```python
from build123d import *

# Parameters (mm, degrees)
BOSS_EXTRUDE1_DEPTH      = 266.7
BOSS_EXTRUDE1_DEPTH_BACK = 266.7
SKETCH3_W                = 25.4
SKETCH3_H                = 25.4
SKETCH3_W_2              = 19.05
SKETCH3_H_2              = 19.05
SKETCH4_R                = 9.525
CUT_EXTRUDE1_DEPTH       = 25.4
SKETCH5_R                = 9.525
CUT_EXTRUDE2_DEPTH       = 3.175


with BuildPart() as part:
    # Sketch3 → Boss-Extrude1 (new, two sides: drawn at the far end of the back side and taken through both)
    with BuildSketch(Plane.XY.offset(-BOSS_EXTRUDE1_DEPTH_BACK)):
        Rectangle(SKETCH3_W, SKETCH3_H)
        Rectangle(SKETCH3_W_2, SKETCH3_H_2, mode=Mode.SUBTRACT)
    extrude(amount=BOSS_EXTRUDE1_DEPTH + BOSS_EXTRUDE1_DEPTH_BACK)

    # Sketch4 → Cut-Extrude1 (cut)
    with BuildSketch(Plane(origin=(0, 12.7, 0), x_dir=(1, 0, 0), z_dir=(0, 1, 0))):
        with Locations(Location((0, 212.725, 0), (0, 0, 180))):
            Circle(SKETCH4_R)
        Polygon((-12.7, 225.013453558), (-12.7, 266.7), (12.7, 266.7), (12.7, 252.73), (-3.69434815, 252.73), align=None)
    extrude(amount=-CUT_EXTRUDE1_DEPTH, mode=Mode.SUBTRACT)

    # Sketch5 → Cut-Extrude2 (cut)
    with BuildSketch(Plane.XZ.offset(-12.7)):
        with Locations(Location((-0.660548484, -179.870948658, 0), (0, 0, 201.463465423))):
            Circle(SKETCH5_R)
    extrude(amount=CUT_EXTRUDE2_DEPTH, mode=Mode.SUBTRACT)


solid = part.part
```
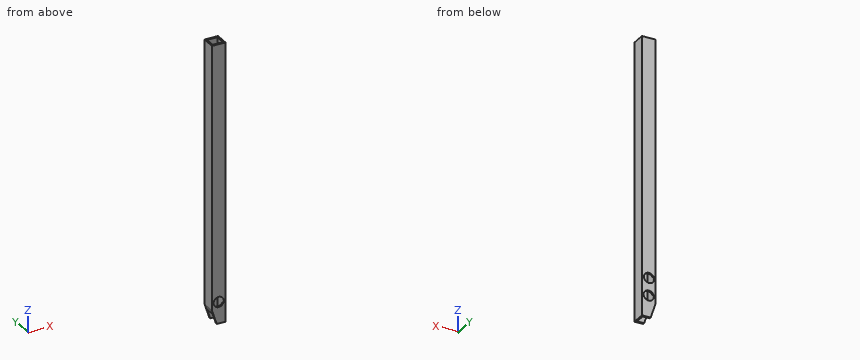
CAD build for the part. Positions are in the model's coordinates, mm. Round coordinates to 2 decimals unless told otherwise and drop trailing zeros. Write each loop counter-clockwise with the first axis right and the second up, starting at its lowest first coordinate (ties: lowest second). Pieces come first, ordered by that corner, then holes.
Item 1: Drill centre lines: L1, parallel to Z at x = 0, y = 11.7; L2, parallel to Y at x = 1, z = 197.5 (3 decimals). Where is each one in solid material? Low to high.
Filled in:
L1: z = -252.73 to -222.25, -203.2 to -189.37, -170.37 to 266.7
L2: y = -12.7 to -9.525, 9.525 to 12.7
Item 2: Band-saw the part on A-A on z = 148. Write the cut outline in (x, y) (3 decimals), then the cut area to 3 significant figures.
Filled in:
outline: (-12.7, -12.7) - (12.7, -12.7) - (12.7, 12.7) - (-12.7, 12.7) - close; hole (-9.525, -9.525) - (9.525, -9.525) - (9.525, 9.525) - (-9.525, 9.525) - close
area: 282 mm2
Item 3: Band-saw the part on B-B on y = 4.75. Write the cut outline in (x, z) (3 decimals).
Filled in:
outline: (-12.7, -225.013) - (-9.525, -234.785) - (-9.525, 266.7) - (-12.7, 266.7) - close; (9.525, -252.73) - (12.7, -252.73) - (12.7, 266.7) - (9.525, 266.7) - close
Item 4: Band-saw the part on D-D on z = -207.5. Write the cut outline in (x, y) (3 decimals).
Filled in:
outline: (-12.7, -12.7) - (-7.964, -12.7) - (-7.964, -9.525) - (-9.525, -9.525) - (-9.525, 9.525) - (-7.964, 9.525) - (-7.964, 12.7) - (-12.7, 12.7) - close; (7.964, -12.7) - (12.7, -12.7) - (12.7, 12.7) - (7.964, 12.7) - (7.964, 9.525) - (9.525, 9.525) - (9.525, -9.525) - (7.964, -9.525) - close
Item 5: Drop flat-ended pins along their axis: pin 1 Ø5 at (x, y) = (-9, -7.5) entering from +Z; pin 2 Ø12 at (x, y) = (1.5, -3) entering from +Z; pin 3 Ø11.5 at (x, z) = (-0.66, -179.87) entering from +Y (3 decimals). Give the stop position or say it passes through.
Filled in:
pin 1: stops at z = 266.7
pin 2: passes through
pin 3: stops at y = -9.525
Item 6: Band-saw the part on C-C on x = 2.75. Write the cut outline in (y, z) (3 decimals).
Filled in:
outline: (-12.7, -252.73) - (-9.525, -252.73) - (-9.525, -221.844) - (-12.7, -221.844) - close; (-12.7, -203.606) - (-9.525, -203.606) - (-9.525, 266.7) - (-12.7, 266.7) - close; (9.525, -252.73) - (12.7, -252.73) - (12.7, -221.844) - (9.525, -221.844) - close; (9.525, -203.606) - (12.7, -203.606) - (12.7, -188.764) - (9.525, -188.764) - close; (9.525, -170.977) - (12.7, -170.977) - (12.7, 266.7) - (9.525, 266.7) - close
